Model file for the job. Use its own axes, mm. A direction names the side the tool comes from. Coordinates: 2 decimals unless noted, no trailing zeros. Loops run counter-clockwise (first coordinate to the right, second up) from the corner with the lowest first, then second, coordinate; pieces in that order, holes last.
from build123d import *

# Parameters (mm, degrees)
SKETCH_2_W                  = 150
SKETCH_2_H                  = 170
EXTRUDE_2_DEPTH             = 170
SHELL_5_T                   = -4
SKETCH_3_W                  = 130
SKETCH_3_H                  = 150
CUT_EXTRUDE_1_DEPTH         = 205.328167417
SKETCH_4_W                  = 150
SKETCH_4_H                  = 170
SKETCH_4_W_2                = 120
SKETCH_4_H_2                = 130
EXTRUDE_3_DEPTH             = 8
EXTRUDE_4_REACH             = 253.843
EXTRUDE_4_DIRECTION_2_DEPTH = 3
SKETCH_6_W                  = 130
SKETCH_6_H                  = 3
CUT_EXTRUDE_2_DEPTH         = 165
FILLET_1_SIZE               = 8


with BuildPart() as part:
    # 草圖2 → 填料-伸長2 (new body)
    with BuildSketch(Plane(origin=(0, 0, 0), x_dir=(1, 0, 0), z_dir=(0, 1, 0))):
        Rectangle(SKETCH_2_W, SKETCH_2_H)
    extrude(amount=EXTRUDE_2_DEPTH)

    # 薄殼5
    shell_5_openings = [part.faces().sort_by_distance(p)[0] for p in [
        (0, 0, 0),
        (0, 85, 85),
    ]]
    offset(amount=SHELL_5_T, openings=shell_5_openings, kind=Kind.INTERSECTION)

    # 草圖3 → 除料-伸長1 (cut, through all)
    with BuildSketch(Plane(origin=(0, 170, 0), x_dir=(1, 0, 0), z_dir=(0, 1, 0))):
        Rectangle(SKETCH_3_W, SKETCH_3_H)
    extrude(amount=-CUT_EXTRUDE_1_DEPTH, mode=Mode.SUBTRACT)

    # 草圖4 → 填料-伸長3 (add)
    with BuildSketch(Plane.XZ.offset(-166)):
        Rectangle(SKETCH_4_W, SKETCH_4_H)
        Rectangle(SKETCH_4_W_2, SKETCH_4_H_2, mode=Mode.SUBTRACT)
    extrude(amount=EXTRUDE_3_DEPTH)

    # 填料-伸長4: up to this face of the body (flat: up to its plane)
    extrude_4_end = Plane(part.part.faces().sort_by_distance((0, 168, 75))[0])
    # 草圖5 → 填料-伸長4 (add, up to the picked face)
    with BuildSketch(Plane.XY.offset(85), mode=Mode.PRIVATE) as extrude_4_sk1:
        Polygon((55, 170), (75, 170), (75, 0), (-75, 0), (-75, 170), (-55, 170), (-55, 15), (55, 15), align=None)
    extrude_4_tool1 = split(extrude(extrude_4_sk1.sketch, amount=-EXTRUDE_4_REACH, mode=Mode.PRIVATE), bisect_by=extrude_4_end, keep=Keep.BOTH, mode=Mode.PRIVATE)
    add(extrude_4_tool1.solids().sort_by(Axis((65, 167.732843, 85), (0, 0, -1)))[0])

    # 草圖5 → 填料-伸長4 direction 2 (add)
    with BuildSketch(Plane.XY.offset(85)):
        Polygon((55, 170), (75, 170), (75, 0), (-75, 0), (-75, 170), (-55, 170), (-55, 15), (55, 15), align=None)
    extrude(amount=EXTRUDE_4_DIRECTION_2_DEPTH)

    # 草圖6 → 除料-伸長2 (cut)
    with BuildSketch(Plane(origin=(0, 170, 0), x_dir=(1, 0, 0), z_dir=(0, 1, 0))):
        with Locations((0, -83.5)):
            Rectangle(SKETCH_6_W, SKETCH_6_H)
    extrude(amount=-CUT_EXTRUDE_2_DEPTH, mode=Mode.SUBTRACT)

    # 圓角1
    # a fillet whose section is not a circle: 8 mm, written as the material it takes off along each edge
    with BuildSketch(Plane(origin=(75, -20, -85), x_dir=(0, 0, 1), z_dir=(0, 1, 0)), Plane(origin=(-75, -20, -85), x_dir=(1, 0, 0), z_dir=(0, 1, 0)), Plane(origin=(75, 190, 88), x_dir=(0, 0, -1), z_dir=(0, -1, 0)), Plane(origin=(-75, -20, 88), x_dir=(0, 0, -1), z_dir=(0, 1, 0))) as fillet_1_piece_1:
        with BuildLine():
            Bezier((FILLET_1_SIZE, 0), (0, 0), (0, -FILLET_1_SIZE), weights=[1, 1, 1])
            Line((0, -FILLET_1_SIZE), (0, 0))
            Line((0, 0), (FILLET_1_SIZE, 0))
        make_face()
    extrude(amount=210, mode=Mode.SUBTRACT)


solid = part.part
Q1. Slice it at A-A (z = -60). List the corners of the cut face in (x, y), and give its area (3 significant figures).
Answers:
outline: (-75, 0) - (-71, 0) - (-71, 158) - (-60, 158) - (-60, 166) - (-65, 166) - (-65, 170) - (-75, 170) - close; (60, 158) - (71, 158) - (71, 0) - (75, 0) - (75, 170) - (65, 170) - (65, 166) - (60, 166) - close
area: 1,580 mm2
Q2. Slice it at C-C (y = 11). Count the separate pieces of the cut face and the enclosed holes in it, and give its area (3 significant figures).
Answers:
separate pieces: 1
enclosed holes: 2
area: 3,370 mm2
Q3. Mould opens along X. For faces 5 (the flat face through (-75, 86, 0)), 6 (the flat face through (0, 10, 88)), 7 (the flat face through (-1, 162, -65)) say: +X half, -X half, draft (parallel to the pull), parting line (faces both ways), or undercut.
Answers:
face 5: -X half
face 6: draft
face 7: undercut
Q4. Flat gauge pins, fed straight in: P1, Ø0.9, axis at x = -19, z = 87, coming from the +Y side; P2, Ø2, axis at x = -30, y = 47.5, coming from the +Z side; P3, Ø1.5, axis at y = 99.5, z = 86, coming from the +X side. Where does each tip first touch, or does it go through?
Answers:
P1: stops at y = 15
P2: stops at z = -81
P3: stops at x = 73.63
Q5. Which spindle directions (+Z, -Z, +X, -X, +Y, -Y) get a long thin tool onto all of the face, cutting with end or side? Do faces 1 (the flat face through (-58, 88, 82)), 2 (the flat face through (55, 85, 78)), 3 (the flat face through (-60, 162, -1)), 4 (the flat face through (71, 78, -2)). Say none if no direction does.
Answers:
face 1: +Y
face 2: +Z
face 3: +Y, -Y
face 4: -Y
Q6. Drill centre lines: line 1 (Z direction, x = -60, y = 55.5); line 2 (X direction, y = 60, z = -50.5); line 3 (X direction, y = 153.5, z = 81). Where is each one in solid material? Low to high.
Answers:
line 1: z = -85 to -81, 75 to 82, 85 to 88
line 2: x = -75 to -71, 71 to 75
line 3: x = -74.97 to -55, 55 to 74.97
Q7. Slice it at B-B (x = -41.5). List the corners of the cut face in (y, z), and give its area (3 significant figures).
Answers:
outline: (0, -85) - (170, -85) - (170, -75) - (166, -75) - (166, -65) - (158, -65) - (158, -81) - (0, -81) - close; (0, 75) - (15, 75) - (15, 82) - (5, 82) - (5, 85) - (15, 85) - (15, 88) - (0, 88) - close; (158, 65) - (166, 65) - (166, 75) - (170, 75) - (170, 82) - (158, 82) - close
area: 1,160 mm2
